Geometry check sheet. Reference: the model listing, model coordinates, mm. A direction names the side the tool comes from. Give positions to 0.01 mm unless a question says otherwise; leave off trailing zeros. Loops run counter-clockwise (first coordinate to the right, second up) from the corner with the lowest first, then second, coordinate; pieces in that order, holes last. Notation, with made-up numbers: (-35.5, 31.5) -> (-27.5, 31.5) arc R19 cw to (-27.5, 40.5) -> close; hole circle Ø6 at (45.5, 64.5). An arc over 180 degrees is marked (long way). One line per item, written item: value. Start each with the question number.
(1) Sectioned sample at A-A, the plane z = 2.05. State how many separate pieces and enclosed holes the cut face has, then the cut area to 3 significant figures.
(2) Sectioned sample at B-B, the plane y = 148.5. Record the cut outline in (x, z).
(3) Tool access check on faces 1 (the face through (28.08, 84.67, 1.48)), 2 (the face through (143, 99, 0)). Record the directions out of +Z, -Z, +X, -X, +Y, -Y that give a thin tool (end or side, any length) a straight path to the whole face; none if there is none.
(4) Draft check along Y on faces 3 (the face through (93.91, 150.47, 1.48)), 4 (the face through (143, 99, 3)), 5 (the face through (32.28, 150.66, 1.48)). Enter one of: pulls with the +Y half, pulls with the -Y half, needs draft (parallel to the pull), parting line crosses it, or undercut.
(5) Scan lines: line 1 along Y through (x, z) = (226, 0.9); line 2 along Y through (x, z) = (25.5, 0.7); line 3 along X through (y, z) = (11.5, 1.5). Record each from-to range of solid material in increasing order. Write a range as from..to.
from build123d import *

# Parameters (mm, degrees)
SKETCH_1_W          = 236
SKETCH_1_H          = 196
SKETCH_1_R          = 2.25
EXTRUDE_1_DEPTH     = 3
SKETCH_2_R          = 1.6
CUT_EXTRUDE_2_DEPTH = 4
FILLET_1_R          = 3


with BuildPart() as part:
    # Эскиз1 → Бобышка-Вытянуть1 (new body)
    with BuildSketch(Plane.XY):
        with Locations((118, 98)):
            Rectangle(SKETCH_1_W, SKETCH_1_H)
        with Locations((10, 183)):
            Circle(SKETCH_1_R, mode=Mode.SUBTRACT)
        with Locations((10, 13)):
            Circle(SKETCH_1_R, mode=Mode.SUBTRACT)
        with Locations((226, 183)):
            Circle(SKETCH_1_R, mode=Mode.SUBTRACT)
        with Locations((226, 13)):
            Circle(SKETCH_1_R, mode=Mode.SUBTRACT)
        with Locations((118, 183)):
            Circle(SKETCH_1_R, mode=Mode.SUBTRACT)
        with Locations((118, 13)):
            Circle(SKETCH_1_R, mode=Mode.SUBTRACT)
    extrude(amount=EXTRUDE_1_DEPTH)

    # Эскиз2 → Вырез-Вытянуть2 (cut, through all)
    with BuildSketch(Plane.XY):
        with Locations((25.5, 52.5)):
            Circle(SKETCH_2_R)
        with Locations((99, 29)):
            Circle(SKETCH_2_R)
        with Locations((35, 167)):
            Circle(SKETCH_2_R)
        with Locations((99, 167)):
            Circle(SKETCH_2_R)
        Polygon((101.75, 142.628747105), (85.878747105, 158.5), (40.121211423, 158.5), (24.25, 142.628788577), (24.25, 88.5), (32, 80.75), (32, 35.5), (42, 25.5), (84, 25.5), (101.75, 43.25), align=None)
    extrude(amount=CUT_EXTRUDE_2_DEPTH, mode=Mode.SUBTRACT)

    # Скругление1
    fillet_1_edges = [part.edges().sort_by_distance(p)[0] for p in [
        (40.121211423, 158.5, 1.5),
        (24.25, 142.628788577, 1.5),
        (24.25, 88.5, 1.5),
        (32, 80.75, 1.5),
        (32, 35.5, 1.5),
        (42, 25.5, 1.5),
        (84, 25.5, 1.5),
        (101.75, 43.25, 1.5),
        (101.75, 142.628747105, 1.5),
        (85.878747105, 158.5, 1.5),
    ]]
    fillet(fillet_1_edges, radius=FILLET_1_R)


solid = part.part
Calculated:
1. separate pieces: 1
1. enclosed holes: 11
1. area: 36,700 mm2
2. outline: (0, 0) -> (30.12, 0) -> (30.12, 3) -> (0, 3) -> close; (95.88, 0) -> (236, 0) -> (236, 3) -> (95.88, 3) -> close
3. face 1: +Z, -Z
3. face 2: -Z, +X, -X, +Y, -Y
4. face 3: undercut
4. face 4: needs draft
4. face 5: undercut
5. line 1: y = 0..10.75, 15.25..180.75, 185.25..196
5. line 2: y = 0..50.9, 54.1..87.25, 143.88..196
5. line 3: x = 0..8.32, 11.68..116.32, 119.68..224.32, 227.68..236
